from build123d import *

# Parameters (mm, degrees)
F1_DEPTH = 25.4
F2_W     = 19.05
F2_H     = 19.05
F3_DEPTH = 650.4296966


with BuildPart() as f1:
    # F0 (on Front) → F1 (new body)
    with BuildSketch(Plane.XZ):
        with BuildLine():
            Line((318.0789541172, -9.1712903899), (-306.9497424828, -9.1712903899))
            Line((-306.9497424828, -9.1712903899), (-306.9497424828, -15.5212903899))
            ThreePointArc((-306.9497424828, -15.5212903899), (-302.4596144223, -17.3811623294), (-300.5997424828, -21.8712903899))
            ThreePointArc((-300.5997424828, -21.8712903899), (-302.4596144223, -26.3614184504), (-306.9497424828, -28.2212903899))
            Line((-306.9497424828, -28.2212903899), (-306.9497424828, -34.5712903899))
            Line((-306.9497424828, -34.5712903899), (318.0789541172, -34.5712903899))
            Line((318.0789541172, -34.5712903899), (318.0789541172, -28.2212903899))
            ThreePointArc((318.0789541172, -28.2212903899), (311.7289541172, -21.8712903899), (318.0789541172, -15.5212903899))
            Line((318.0789541172, -15.5212903899), (318.0789541172, -9.1712903899))
        make_face()
        with BuildLine():
            Line((-306.9497424828, -15.5212903899), (-306.9497424828, -9.1712903899))
            ThreePointArc((-306.9497424828, -9.1712903899), (-315.9299986039, -12.8910342688), (-319.6497424828, -21.8712903899))
            ThreePointArc((-319.6497424828, -21.8712903899), (-315.9299986039, -30.851546511), (-306.9497424828, -34.5712903899))
            Line((-306.9497424828, -34.5712903899), (-306.9497424828, -28.2212903899))
            ThreePointArc((-306.9497424828, -28.2212903899), (-313.2997424828, -21.8712903899), (-306.9497424828, -15.5212903899))
        make_face()
        with BuildLine():
            Line((330.7789541172, -9.1712903899), (318.0789541172, -9.1712903899))
            ThreePointArc((318.0789541172, -9.1712903899), (327.0592102383, -12.8910342688), (330.7789541172, -21.8712903899))
            Line((330.7789541172, -21.8712903899), (330.7789541172, -9.1712903899))
        make_face()
        with BuildLine():
            Line((330.7789541172, -34.5712903899), (330.7789541172, -21.8712903899))
            ThreePointArc((330.7789541172, -21.8712903899), (327.0592102383, -30.851546511), (318.0789541172, -34.5712903899))
            Line((318.0789541172, -34.5712903899), (330.7789541172, -34.5712903899))
        make_face()
        with BuildLine():
            ThreePointArc((330.7789541172, -21.8712903899), (327.0592102383, -12.8910342688), (318.0789541172, -9.1712903899))
            Line((318.0789541172, -9.1712903899), (318.0789541172, -15.5212903899))
            ThreePointArc((318.0789541172, -15.5212903899), (322.5690821777, -17.3811623294), (324.4289541172, -21.8712903899))
            ThreePointArc((324.4289541172, -21.8712903899), (322.5690821777, -26.3614184504), (318.0789541172, -28.2212903899))
            Line((318.0789541172, -28.2212903899), (318.0789541172, -34.5712903899))
            ThreePointArc((318.0789541172, -34.5712903899), (327.0592102383, -30.851546511), (330.7789541172, -21.8712903899))
        make_face()
        with BuildLine():
            ThreePointArc((-319.6497424828, -21.8712903899), (-315.9299986039, -12.8910342688), (-306.9497424828, -9.1712903899))
            Line((-306.9497424828, -9.1712903899), (-319.6497424828, -9.1712903899))
            Line((-319.6497424828, -9.1712903899), (-319.6497424828, -21.8712903899))
        make_face()
        with BuildLine():
            ThreePointArc((-306.9497424828, -34.5712903899), (-315.9299986039, -30.851546511), (-319.6497424828, -21.8712903899))
            Line((-319.6497424828, -21.8712903899), (-319.6497424828, -34.5712903899))
            Line((-319.6497424828, -34.5712903899), (-306.9497424828, -34.5712903899))
        make_face()
    extrude(amount=F1_DEPTH)

    # F2 (on face) → F3 (cut, through all)
    with BuildSketch(Plane(origin=(-319.6497424828, 0, 0), x_dir=(0, -1, 0), z_dir=(-1, 0, 0))):
        with Locations((12.7, -21.8712903899)):
            Rectangle(F2_W, F2_H)
    extrude(amount=-F3_DEPTH, mode=Mode.SUBTRACT)


solid = f1.part
Check sheet for the modelled part. Datum: model origin and axes. Units: mm. A direction names the side the tool comes from. Coordinates: 2 decimals unless noted, no trailing zeros. Loops run counter-clockwise (first coordinate to the right, second up) from the corner with the lowest first, then second, coordinate; pieces in that order, holes last. Notation, with made-up numbers: (-0.75, 40.5) -> (44.25, 40.5) arc R24 ccw to (44.25, 77.5) -> close; hole circle Ø9 at (0.5, -38). An arc over 180 degrees is marked (long way). Answer in a Markdown table with one row per item.
1. Sectioned sample at B-B, the plane x = 156.5. Record the boundary of the cut face in (y, z) (3 decimals).
Check values:
| item | result |
|---|---|
| outline | (-25.4, -34.571) -> (0, -34.571) -> (0, -9.171) -> (-25.4, -9.171) -> close; hole (-22.225, -31.396) -> (-3.175, -31.396) -> (-3.175, -12.346) -> (-22.225, -12.346) -> close |
2. Release check for a two-part mould opening along Z. For faces 3 (the face through (1, -13, -31.396)), 4 (the face through (1, -13, -34.571)), 5 (the face through (330.779, -13, -33)), 6 (the face through (10, -13, -9.171)) record: released by +Z, released by -Z, zero draft, split by the parting line, or undercut.
Check values:
| item | result |
|---|---|
| face 3 | undercut |
| face 4 | released by -Z |
| face 5 | zero draft |
| face 6 | released by +Z |
3. Go/stop test with a flat-tipped pin: pin 1 (8 mm diameter, centred on x = 186.5, z = -20.5, fed in from +Y). Record where the tip stops, or that it passes through.
Check values:
| item | result |
|---|---|
| pin 1 | stops at y = 0 |
4. Sectioned sample at A-A, the plane y = -9. Record the boundary of the cut face in (x, z).
Check values:
| item | result |
|---|---|
| outline | (-319.65, -34.57) -> (330.78, -34.57) -> (330.78, -31.4) -> (-319.65, -31.4) -> close; (-319.65, -12.35) -> (330.78, -12.35) -> (330.78, -9.17) -> (-319.65, -9.17) -> close |
5. Access from +Z, -Z, +X, -X, +Y, -Y to the whole of each face (thin tool, end or side, straight path). Record for faces 1 (the face through (-319.65, -13, -33)), 2 (the face through (1, -3.175, -22)).
Check values:
| item | result |
|---|---|
| face 1 | +Z, -Z, -X, +Y, -Y |
| face 2 | +X, -X |
6. Material ranges on line 1 along Z through (x, y) = (83, -8.5); line 2 along Y through (x, z) = (-260, -29.25) (3 decimals); line 3 along X through (y, z) = (-2.5, -17.75), recorded low to high. Write a range as [from, to].
Check values:
| item | result |
|---|---|
| line 1 | z = [-34.57, -31.4], [-12.35, -9.17] |
| line 2 | y = [-25.4, -22.225], [-3.175, 0] |
| line 3 | x = [-319.65, -311.78], [-302.12, 313.25], [322.91, 330.78] |
